The model under review builds one solid part; all positions refer to its coordinate system, in mm. A direction names the side the tool comes from. Round coordinates to 2 decimals unless told otherwise and drop trailing zeros. Write each loop counter-clockwise with the first axis right and the second up, starting at its lowest first coordinate (ties: lowest second). Pieces come first, ordered by that corner, then holes. Notation, with made-up numbers: M -39,15 L 8,15 A28 ccw 8,51 Z; hole C 38.25,-32.5 d4. An arc over 180 degrees is marked long. Write item = value, one per line. Start each with the question number.
Item 1: The part is to be moulded in two halves that separate along Y. For faces 1 (the flat face through (-23.79, -3.48, -12.05)), 2 (the conical face through (-65.9, -7.8, 29.4)), 3 (the flat face through (0, -29, 18)), say which applies: +Y half, -Y half, draft (parallel to the pull), parting line (faces both ways), or undercut.
Item 2: Tool access review of faces 4 (the cylindrical face through (-55.104, -10.474, 20.452)), 5 (the flat face through (24.28, -3.48, -11.56)): name each direction out of +Z, -Z, +X, -X, +Y, -Y from which nothing blocks a thin tool from reaching the whole face with its end or side.
Item 3: For pin 1 Ø4.5 at (x, z) = (48, 3.78) entering from +Y; pin 2 Ø12 at (x, y) = (31.5, -11) entering from +Z; pin 3 Ø2 at (x, y) = (-48.5, -23.5) entering from -Z; pin 4 Ø12 at (y, z) = (-11, 20) entering from -X, all flat-tipped, find the tip position at first contact; note any pin that passes through.
Item 4: Take a section at A-A, the plane x = -20.5. Give the boundary of the cut face in (y, z).
Item 5: To check wall thickness, follow line 1 along X through (y, z) = (-19, 21.5); line 2 along Z through (x, y) = (22.5, -9.75); line 3 along Z through (x, y) = (-35, -21.25). State the ranges of each line that lie inside material, in increasing order.
from build123d import *

# Parameters (mm, degrees)
SKETCH_1_R                   = 2
SKETCH_1_R_2                 = 1
EXTRUDE_1_DEPTH              = 29
CUT_EXTRUDE_1_DEPTH          = 5
CUT_EXTRUDE_START            = -10
CUT_EXTRUDE_2_DEPTH          = 19
CUT_EXTRUDE_3_DEPTH          = 2
SKETCH_11_R                  = 1.6
CUT_EXTRUDE_4_DEPTH          = 104.437531222
SKETCH_13_R                  = 1.25
CUT_EXTRUDE_5_DEPTH          = 2
HOLE_WIZARD_M2_5_6_D         = 2.05
HOLE_WIZARD_M3_1_D           = 2.5
HOLE_WIZARD_M3_1_CSINK_D     = 3.05
HOLE_WIZARD_M3_1_CSINK_ANGLE = 90
CHAMFER_1_SIZE               = 2
FILLET_1_R                   = 3
CHAMFER_2_SIZE               = 1.65


with BuildPart() as part:
    # Sketch 1 → Extrude 1 (new body)
    # profile 1 of 2: a face of its own
    with BuildSketch(Plane(origin=(0, 0, 0), x_dir=(1, 0, 0), z_dir=(0, 1, 0))):
        Polygon((69.296464556, -30.626082539), (66.468037432, -33.454509664), (51.618795027, -18.605267259), (47.376154339, -22.847907946), (43.376154339, -22.847907946), (39.133513652, -18.605267259), (0.638005734, -18.605267259), (-39.133513652, -18.605267259), (-43.376154339, -22.847907946), (-47.376154339, -22.847907946), (-51.618795027, -18.605267259), (-66.468037432, -33.454509664), (-69.296464556, -30.626082539), (-53.656854249, -14.986472232), (-53.656854249, -3.776840134), (-28, 21.880014115), (-16.790367902, 21.880014115), (0, 38.670382017), (16.790367902, 21.880014115), (28, 21.880014115), (53.656854249, -3.776840134), (53.656854249, -14.986472232), align=None)
        with Locations(Location((28, 16.223159866, 0), (0, 0, 270))):
            Circle(SKETCH_1_R, mode=Mode.SUBTRACT)
        with Locations(Location((-28, 16.223159866, 0), (0, 0, 270))):
            Circle(SKETCH_1_R, mode=Mode.SUBTRACT)
        with Locations(Location((-48, -3.776840134, 0), (0, 0, 270))):
            Circle(SKETCH_1_R, mode=Mode.SUBTRACT)
        with Locations(Location((44.194173824, -11.180646057, 0), (0, 0, 270))):
            Circle(SKETCH_1_R_2, mode=Mode.SUBTRACT)
        with Locations(Location((-44.194173824, -11.180646057, 0), (0, 0, 270))):
            Circle(SKETCH_1_R_2, mode=Mode.SUBTRACT)
        with Locations(Location((0, 33.013527768, 0), (0, 0, 270))):
            Circle(SKETCH_1_R_2, mode=Mode.SUBTRACT)
        with Locations(Location((48, -3.776840134, 0), (0, 0, 270))):
            Circle(SKETCH_1_R, mode=Mode.SUBTRACT)
        Polygon((-43.487067043, -7.645112151), (-37.355339059, -13.776840134), (37.355339059, -13.776840134), (43.487067043, -7.645112151), (5.828427125, 30.013527768), (-5.828427125, 30.013527768), align=None, mode=Mode.SUBTRACT)
    # profile 2 of 2: a face of its own
    with BuildSketch(Plane(origin=(0, 0, 0), x_dir=(1, 0, 0), z_dir=(0, 1, 0))):
        Polygon((-5.828427125, 30.013527768), (-43.487067043, -7.645112151), (-37.355339059, -13.776840134), (37.355339059, -13.776840134), (43.487067043, -7.645112151), (5.828427125, 30.013527768), align=None)
    extrude(amount=-EXTRUDE_1_DEPTH)

    # Sketch 1_3 → Cut-Extrude 1 (cut)
    with BuildSketch(Plane(origin=(0, 0, 0), x_dir=(1, 0, 0), z_dir=(0, 1, 0))):
        Polygon((-5.828427125, 30.013527768), (-43.487067043, -7.645112151), (-37.355339059, -13.776840134), (37.355339059, -13.776840134), (43.487067043, -7.645112151), (5.828427125, 30.013527768), align=None)
    extrude(amount=-CUT_EXTRUDE_1_DEPTH, mode=Mode.SUBTRACT)

    # Sketch 3 → Cut-Extrude 2 (cut)
    with BuildSketch(Plane(origin=(0, 0, 0), x_dir=(1, 0, 0), z_dir=(0, 1, 0)).offset(CUT_EXTRUDE_START)):
        Polygon((-74.127206293, -13.776840134), (70.632375227, -13.776840134), (4.598461929, 56.317971506), align=None)
    extrude(amount=-CUT_EXTRUDE_2_DEPTH, mode=Mode.SUBTRACT)

    # Sketch 4 → Cut-Extrude 3 (cut)
    with BuildSketch(Plane(origin=(0, 0, 0), x_dir=(1, 0, 0), z_dir=(0, 1, 0))):
        with BuildLine():
            Line((-2.121320344, 36.549061673), (-48.535533906, -9.865151889))
            ThreePointArc((-48.535533906, -9.865151889), (-49.18585216, -13.13452253), (-46.414213562, -14.986472232))
            Line((-46.414213562, -14.986472232), (46.414213562, -14.986472232))
            ThreePointArc((46.414213562, -14.986472232), (49.18585216, -13.13452253), (48.535533906, -9.865151889))
            Line((48.535533906, -9.865151889), (0, 38.670382017))
            Line((0, 38.670382017), (-2.121320344, 36.549061673))
        make_face()
    extrude(amount=-CUT_EXTRUDE_3_DEPTH, mode=Mode.SUBTRACT)

    # Sketch 11 → Cut-Extrude 4 (cut, through all)
    with BuildSketch(Plane(origin=(-16.506763884, 0, -16.506763884), x_dir=(0.7071067811865477, 0, -0.7071067811865474), z_dir=(0.7071067811865474, 0, 0.7071067811865477))):
        with Locations((-52.155910645, -9.5)):
            Circle(SKETCH_11_R)
        with Locations((-52.155910645, -19.5)):
            Circle(SKETCH_11_R)
        with Locations((-67.155910645, -19.5)):
            Circle(SKETCH_11_R)
        with Locations((-67.155910645, -9.5)):
            Circle(SKETCH_11_R)
    cut_extrude_4 = extrude(amount=-CUT_EXTRUDE_4_DEPTH, mode=Mode.SUBTRACT)

    # Sketch 13 → Cut-Extrude 5 (cut)
    with BuildSketch(Plane(origin=(-19.335191009, 0, -19.335191009), x_dir=(-0.7071067811865488, 0, 0.7071067811865462), z_dir=(-0.7071067811865462, 0, -0.7071067811865488))):
        with Locations((59.597036142, -26)):
            Circle(SKETCH_13_R)
    cut_extrude_5 = extrude(amount=-CUT_EXTRUDE_5_DEPTH, mode=Mode.SUBTRACT)

    # Hole Wizard M2.5 _6 (through all)
    with Locations(Plane(origin=(0, -2, -33.013527768), x_dir=(0, 0, 1), z_dir=(0, 1, 0))):
        with Locations((0, 0), (44.194173825, -44.194173824), (44.194173825, 44.194173824)):
            Hole(HOLE_WIZARD_M2_5_6_D / 2)

    # Hole Wizard M3 _1 (through all)
    with Locations(Plane(origin=(-61.476659403, -26, 22.806277386), x_dir=(-0.707106781187, 0, 0.707106781187), z_dir=(-0.707106781187, 0, -0.707106781187))):
        with Locations((0, 0)):
            hole_wizard_m3_1 = CounterSinkHole(HOLE_WIZARD_M3_1_D / 2, HOLE_WIZARD_M3_1_CSINK_D / 2, counter_sink_angle=HOLE_WIZARD_M3_1_CSINK_ANGLE)

    # Mirror 2: Cut-Extrude 4, Cut-Extrude 5, Hole Wizard M3 _1 across plane
    add(cut_extrude_4.mirror(Plane.ZY), mode=Mode.SUBTRACT)
    add(cut_extrude_5.mirror(Plane.ZY), mode=Mode.SUBTRACT)
    add(hole_wizard_m3_1.mirror(Plane.ZY), mode=Mode.SUBTRACT)

    # Chamfer 1
    chamfer_1_edges = [part.edges().sort_by_distance(p)[0] for p in [
        (0, -6, -38.670382017),
    ]]
    chamfer(chamfer_1_edges, length=CHAMFER_1_SIZE)

    # Fillet 1
    fillet_1_edges = [part.edges().sort_by_distance(p)[0] for p in [
        (16.790367902, -6, -21.880014115),
        (-16.790367902, -6, -21.880014115),
        (39.133513652, -14.5, 18.605267259),
        (-39.133513652, -14.5, 18.605267259),
        (-43.487067043, -3.5, 7.645112151),
        (-5.828427125, -3.5, -30.013527768),
        (5.828427125, -3.5, -30.013527768),
        (43.487067043, -3.5, 7.645112151),
        (37.355339059, -3.5, 13.776840134),
        (-37.355339059, -3.5, 13.776840134),
    ]]
    fillet(fillet_1_edges, radius=FILLET_1_R)

    # Chamfer 2
    chamfer_2_edges = [part.edges().sort_by_distance(p)[0] for p in [
        (-67.952961672, -9.5, 29.282579655),
        (-57.346359954, -19.5, 18.675977937),
        (-67.952961672, -19.5, 29.282579655),
        (-57.346359954, -9.5, 18.675977937),
        (67.952961672, -9.5, 29.282579655),
        (57.346359954, -19.5, 18.675977937),
        (67.952961672, -19.5, 29.282579655),
        (57.346359954, -9.5, 18.675977937),
    ]]
    chamfer(chamfer_2_edges, length=CHAMFER_2_SIZE)


solid = part.part
Response values:
q1.face_1 = draft
q1.face_2 = undercut
q1.face_3 = -Y half
q2.face_4 = none
q2.face_5 = +Y
q3.pin_1 = 0
q3.pin_2 = 18.61
q3.pin_3 = 13.78
q3.pin_4 = -64.67
q4.outline = M -29,13.78 L -10,13.78 L -10,-21.88 L 0,-21.88 L 0,-18.17 L -2,-18.17 L -2,-15.34 L -5,-15.34 L -5,13.78 L -2,13.78 L -2,14.99 L 0,14.99 L 0,18.61 L -29,18.61 Z
q5.line_1 = -60.17 to -54.51, -48.72 to -42.03, 42.03 to 48.72, 54.51 to 60.17
q5.line_2 = -21.88 to 18.61
q5.line_3 = 13.78 to 18.61
